from build123d import *

# Parameters (mm, degrees)
BOSS_EXTRUDE1_DEPTH              = 4.763
TAP_DRILL_FOR_M3X0_5_TAP1_REACH  = 220.74
TAP_DRILL_FOR_M3X0_5_TAP1_BORE_R = 1.25
TAP_DRILL_FOR_M3X0_5_TAP2_REACH  = 220.74
TAP_DRILL_FOR_M3X0_5_TAP2_BORE_R = 1.25


with BuildPart() as part:
    # Sketch3 → Boss-Extrude1 (new body)
    with BuildSketch(Plane.XY):
        Polygon((-108.762998674, 22.483018567), (-108.762998674, -22.516981433), (-103.762998674, -22.516981433), (-45, -11.683163514), (45, -11.683163514), (103.762998674, -22.483018567), (108.762998674, -22.483018567), (108.762998674, 22.516981433), (103.762998674, 22.516981433), (45, 11.683163514), (-45, 11.683163514), (-103.762998674, 22.483018567), align=None)
        with BuildLine():
            Line((-45, -3.923438204), (45, -3.923438204))
            ThreePointArc((45, -3.923438204), (46.379862655, -5.303300859), (45, -6.683163514))
            Line((45, -6.683163514), (-45, -6.683163514))
            ThreePointArc((-45, -6.683163514), (-46.379862655, -5.303300859), (-45, -3.923438204))
        make_face(mode=Mode.SUBTRACT)
        with BuildLine():
            Line((-45, 6.683163514), (45, 6.683163514))
            ThreePointArc((45, 6.683163514), (46.379862655, 5.303300859), (45, 3.923438204))
            Line((45, 3.923438204), (-45, 3.923438204))
            ThreePointArc((-45, 3.923438204), (-46.379862655, 5.303300859), (-45, 6.683163514))
        make_face(mode=Mode.SUBTRACT)
        with BuildLine():
            Line((-103.762998674, 15.571322269), (-103.762998674, 4.07129926))
            ThreePointArc((-103.762998674, 4.07129926), (-103.298030689, 2.948767244), (-102.175498674, 2.48379926))
            Line((-102.175498674, 2.48379926), (-78.468999337, 2.48379926))
            ThreePointArc((-78.468999337, 2.48379926), (-77.346467322, 2.948767244), (-76.881499337, 4.07129926))
            Line((-76.881499337, 4.07129926), (-76.881499337, 11.140532377))
            ThreePointArc((-76.881499337, 11.140532377), (-77.247696598, 12.154719672), (-78.177342953, 12.701010766))
            Line((-78.177342953, 12.701010766), (-101.88384229, 17.131800658))
            ThreePointArc((-101.88384229, 17.131800658), (-103.18968597, 16.792625008), (-103.762998674, 15.571322269))
        make_face(mode=Mode.SUBTRACT)
        with BuildLine():
            Line((-52.721922194, -8.035531504), (-70.003544755, -11.217242177))
            ThreePointArc((-70.003544755, -11.217242177), (-71.306631893, -10.87607345), (-71.878487463, -9.656477863))
            Line((-71.878487463, -9.656477863), (-71.880224509, -4.093745129))
            ThreePointArc((-71.880224509, -4.093745129), (-71.415607074, -2.971067976), (-70.293220307, -2.505749486))
            Line((-70.293220307, -2.505749486), (-52.984228369, -2.500344496))
            ThreePointArc((-52.984228369, -2.500344496), (-51.855362923, -2.971180632), (-51.396324213, -4.104894584))
            Line((-51.396324213, -4.104894584), (-51.421956543, -6.491321636))
            ThreePointArc((-51.421956543, -6.491321636), (-51.794905097, -7.496642951), (-52.721922194, -8.035531504))
        make_face(mode=Mode.SUBTRACT)
        with BuildLine():
            Line((-71.881499337, 9.634032264), (-71.881499337, 4.07129926))
            ThreePointArc((-71.881499337, 4.07129926), (-71.416531352, 2.948767244), (-70.293999337, 2.48379926))
            Line((-70.293999337, 2.48379926), (-52.985006556, 2.48379926))
            ThreePointArc((-52.985006556, 2.48379926), (-51.85628819, 2.954987878), (-51.397603521, 4.088845117))
            Line((-51.397603521, 4.088845117), (-51.423981048, 6.475264048))
            ThreePointArc((-51.423981048, 6.475264048), (-51.79724351, 7.480468855), (-52.724428838, 8.019067907))
            Line((-52.724428838, 8.019067907), (-70.007044093, 11.195381981))
            ThreePointArc((-70.007044093, 11.195381981), (-71.310024632, 10.853806362), (-71.881499337, 9.634032264))
        make_face(mode=Mode.SUBTRACT)
        with BuildLine():
            Line((-78.468219908, -2.508302252), (-102.17471809, -2.515704959))
            ThreePointArc((-102.17471809, -2.515704959), (-103.297104857, -2.981023449), (-103.761722292, -4.103700602))
            Line((-103.761722292, -4.103700602), (-103.758131238, -15.603723051))
            ThreePointArc((-103.758131238, -15.603723051), (-103.184437192, -16.824846705), (-101.878487663, -17.16361457))
            Line((-101.878487663, -17.16361457), (-78.173373062, -12.725422186))
            ThreePointArc((-78.173373062, -12.725422186), (-77.24389734, -12.178840823), (-76.878016792, -11.164539226))
            Line((-76.878016792, -11.164539226), (-76.880224265, -4.095306454))
            ThreePointArc((-76.880224265, -4.095306454), (-77.345542755, -2.972919687), (-78.468219908, -2.508302252))
        make_face(mode=Mode.SUBTRACT)
        with BuildLine():
            Line((103.758131238, -15.603723051), (103.761722292, -4.103700602))
            ThreePointArc((103.761722292, -4.103700602), (103.297104857, -2.981023449), (102.17471809, -2.515704959))
            Line((102.17471809, -2.515704959), (78.468219908, -2.508302252))
            ThreePointArc((78.468219908, -2.508302252), (77.345542755, -2.972919687), (76.880224265, -4.095306454))
            Line((76.880224265, -4.095306454), (76.878016792, -11.164539226))
            ThreePointArc((76.878016792, -11.164539226), (77.24389734, -12.178840823), (78.173373062, -12.725422186))
            Line((78.173373062, -12.725422186), (101.878487663, -17.16361457))
            ThreePointArc((101.878487663, -17.16361457), (103.184437192, -16.824846705), (103.758131238, -15.603723051))
        make_face(mode=Mode.SUBTRACT)
        with BuildLine():
            Line((71.878487463, -9.656477863), (71.880224509, -4.093745129))
            ThreePointArc((71.880224509, -4.093745129), (71.415607074, -2.971067976), (70.293220307, -2.505749486))
            Line((70.293220307, -2.505749486), (52.984228369, -2.500344496))
            ThreePointArc((52.984228369, -2.500344496), (51.855362923, -2.971180632), (51.396324213, -4.104894584))
            Line((51.396324213, -4.104894584), (51.421956543, -6.491321636))
            ThreePointArc((51.421956543, -6.491321636), (51.794905097, -7.496642951), (52.721922194, -8.035531504))
            Line((52.721922194, -8.035531504), (70.003544755, -11.217242177))
            ThreePointArc((70.003544755, -11.217242177), (71.306631893, -10.87607345), (71.878487463, -9.656477863))
        make_face(mode=Mode.SUBTRACT)
        with BuildLine():
            Line((52.719410409, 8.051994317), (70.000038591, 11.239101279))
            ThreePointArc((70.000038591, 11.239101279), (71.3032322, 10.898339477), (71.875468579, 9.67892252))
            Line((71.875468579, 9.67892252), (71.878942671, 4.1161906))
            ThreePointArc((71.878942671, 4.1161906), (71.414675832, 2.993368417), (70.292434422, 2.527699469))
            Line((70.292434422, 2.527699469), (52.983445016, 2.516889488))
            ThreePointArc((52.983445016, 2.516889488), (51.854432599, 2.987373096), (51.395039893, 4.120943651))
            Line((51.395039893, 4.120943651), (51.419927024, 6.507378591))
            ThreePointArc((51.419927024, 6.507378591), (51.792561634, 7.512816316), (52.719410409, 8.051994317))
        make_face(mode=Mode.SUBTRACT)
        with BuildLine():
            Line((78.467432828, 2.532804999), (102.173927542, 2.547610413))
            ThreePointArc((102.173927542, 2.547610413), (103.296168952, 3.013279362), (103.760435791, 4.136101544))
            Line((103.760435791, 4.136101544), (103.753253685, 15.636122311))
            ThreePointArc((103.753253685, 15.636122311), (103.179178352, 16.857066761), (101.873123102, 17.195426807))
            Line((101.873123102, 17.195426807), (78.169395548, 12.749832365))
            ThreePointArc((78.169395548, 12.749832365), (77.24009055, 12.202960786), (76.87452675, 11.188544987))
            Line((76.87452675, 11.188544987), (76.878941696, 4.119313249))
            ThreePointArc((76.878941696, 4.119313249), (77.344610645, 2.997071839), (78.467432828, 2.532804999))
        make_face(mode=Mode.SUBTRACT)
    extrude(amount=BOSS_EXTRUDE1_DEPTH)

    # Tap Drill for M3x0.5 Tap1 bore → Tap Drill for M3x0.5 Tap1 (cut, up to next)
    with BuildSketch(Plane(origin=(108.762998674, 0, 0), x_dir=(0, 0, -1), z_dir=(1, 0, 0)), mode=Mode.PRIVATE) as tap_drill_for_m3x0_5_tap1_sk1:
        with Locations((-2.3815, 11.266981433)):
            Circle(TAP_DRILL_FOR_M3X0_5_TAP1_BORE_R)
    tap_drill_for_m3x0_5_tap1_tool1 = extrude(tap_drill_for_m3x0_5_tap1_sk1.sketch, amount=-TAP_DRILL_FOR_M3X0_5_TAP1_REACH, mode=Mode.PRIVATE) & part.part
    # Tap Drill for M3x0.5 Tap1 bore → Tap Drill for M3x0.5 Tap1 (cut, up to next)
    with BuildSketch(Plane(origin=(108.762998674, 0, 0), x_dir=(0, 0, -1), z_dir=(1, 0, 0)), mode=Mode.PRIVATE) as tap_drill_for_m3x0_5_tap1_sk2:
        with Locations((-2.3815, -11.233018567)):
            Circle(TAP_DRILL_FOR_M3X0_5_TAP1_BORE_R)
    tap_drill_for_m3x0_5_tap1_tool2 = extrude(tap_drill_for_m3x0_5_tap1_sk2.sketch, amount=-TAP_DRILL_FOR_M3X0_5_TAP1_REACH, mode=Mode.PRIVATE) & part.part
    add(tap_drill_for_m3x0_5_tap1_tool1.solids().sort_by_distance((108.762999, 11.266981, 2.3815))[0], mode=Mode.SUBTRACT)
    add(tap_drill_for_m3x0_5_tap1_tool2.solids().sort_by_distance((108.762999, -11.233019, 2.3815))[0], mode=Mode.SUBTRACT)

    # Tap Drill for M3x0.5 Tap2 bore → Tap Drill for M3x0.5 Tap2 (cut, up to next)
    with BuildSketch(Plane.ZY.offset(108.762998674), mode=Mode.PRIVATE) as tap_drill_for_m3x0_5_tap2_sk1:
        with Locations((2.3815, 11.233018567)):
            Circle(TAP_DRILL_FOR_M3X0_5_TAP2_BORE_R)
    tap_drill_for_m3x0_5_tap2_tool1 = extrude(tap_drill_for_m3x0_5_tap2_sk1.sketch, amount=-TAP_DRILL_FOR_M3X0_5_TAP2_REACH, mode=Mode.PRIVATE) & part.part
    # Tap Drill for M3x0.5 Tap2 bore → Tap Drill for M3x0.5 Tap2 (cut, up to next)
    with BuildSketch(Plane.ZY.offset(108.762998674), mode=Mode.PRIVATE) as tap_drill_for_m3x0_5_tap2_sk2:
        with Locations((2.3815, -11.266981433)):
            Circle(TAP_DRILL_FOR_M3X0_5_TAP2_BORE_R)
    tap_drill_for_m3x0_5_tap2_tool2 = extrude(tap_drill_for_m3x0_5_tap2_sk2.sketch, amount=-TAP_DRILL_FOR_M3X0_5_TAP2_REACH, mode=Mode.PRIVATE) & part.part
    add(tap_drill_for_m3x0_5_tap2_tool1.solids().sort_by_distance((-108.762999, 11.233019, 2.3815))[0], mode=Mode.SUBTRACT)
    add(tap_drill_for_m3x0_5_tap2_tool2.solids().sort_by_distance((-108.762999, -11.266981, 2.3815))[0], mode=Mode.SUBTRACT)


solid = part.part
Read the model definition and answer for the solid it produces. Units are mm, in the model's axes. A direction names the side the tool comes from. Coordinates: 2 decimals unless noted, no trailing zeros. Loops run counter-clockwise (first coordinate to the right, second up) from the corner with the lowest first, then second, coordinate; pieces in that order, holes last.
Q1. Each of these flat-tipped pins is pushed along its axis until it touches: pin 1 Ø2.5 at (x, z) = (63.5, 2) entering from -Y; pin 2 Ø1.4 at (x, z) = (15, 1.5) entering from -Y; pin 3 Ø1.5 at (y, z) = (11.23, 2.38) entering from +X. Where does it stop, or does it pass through?
Q2. Consider probe 1 along Y at (x, z) = (15.5, 1.05); probe 2 along Y at (x, z) = (-57, 3); probe 3 along X at (y, z) = (4.5, 3.8). Determine where each line is inside the solid, lowest interval first.
Q3. The part is cut by section B-B on x = 64.5. Write down the section's boundary in (y, z), and give its area (3 significant figures).
Q4. The part is cut by section C-C on z = 2.85. Give the number of separate pieces and of enclosed holes in the cut face, and give its area (3 significant figures).
Q5. The mould has two halves that part along Y. Classify faces 4 (the face through (-90.192, -14.976, 2.348)), 5 (the face through (106, 22.517, 2)), 6 (the face through (-106, -22.517, 2)): +Y half, -Y half, draft (parallel to the pull), parting line (faces both ways), or undercut.
Q6. Which of the six approach directions +Z, -Z, +X, -X, +Y, -Y give full straight-line access (tool end or side, diameter ignored) to faces 1 (the face through (-61.242, -9.604, 2.348)), 2 (the face through (-74.793, -17.176, 2.348)), 3 (the face through (-2, 0, 4.763))?
Q7. The part is cut by section A-A on x = 39.5. Write down the section's boundary in (y, z).
Results below:
1. pin 1: stops at y = -15.31
1. pin 2: stops at y = -11.68
1. pin 3: stops at x = 77.09
2. probe 1: y = -11.68 to -6.68, -3.92 to 3.92, 6.68 to 11.68
2. probe 2: y = -13.9 to -8.82, -2.5 to 2.48, 8.8 to 13.89
2. probe 3: x = -108.76 to -103.76, -76.88 to -71.88, -51.4 to -46.12, 46.12 to 51.4, 71.88 to 76.88, 103.76 to 108.76
3. outline: (-15.27, 0) - (-10.2, 0) - (-10.2, 4.76) - (-15.27, 4.76) - close; (-2.5, 0) - (2.52, 0) - (2.52, 4.76) - (-2.5, 4.76) - close; (10.22, 0) - (15.28, 0) - (15.28, 4.76) - (10.22, 4.76) - close
3. area: 72.1 mm2
4. separate pieces: 1
4. enclosed holes: 6
4. area: 4,100 mm2
5. face 4: undercut
5. face 5: +Y half
5. face 6: -Y half
6. face 1: +Z, -Z
6. face 2: +Z, -Z, -Y
6. face 3: +Z, +X, -X, +Y, -Y
7. outline: (-11.68, 0) - (-6.68, 0) - (-6.68, 4.76) - (-11.68, 4.76) - close; (-3.92, 0) - (3.92, 0) - (3.92, 4.76) - (-3.92, 4.76) - close; (6.68, 0) - (11.68, 0) - (11.68, 4.76) - (6.68, 4.76) - close
